The model under review builds one solid part; all positions refer to its coordinate system, in mm. A direction names the side the tool comes from. Coordinates: 2 decimals unless noted, no trailing zeros. Order: outer loops, then holes, each group sorted by start corner. A loop starts at its lowest first (then second) coordinate and runs counter-clockwise, first axis right, second up. Notation, with made-up numbers: (59, 7) -> (77, 7) arc R21 ccw to (77, 17) -> close; hole circle Ø9 at (86.25, 51). An arc over 180 degrees is marked (long way). Use one line per item in the form item = value. Start each with the question number.
(1) Take a section at B-B (x = 17.25). State the section outline as (y, z) points, then the cut area to 3 significant figures.
(2) Mouldability with a two-part tool opening along Y and no side actions: class faces 5 (the flat face through (5.5, 0, 22)), 6 (the flat face through (11, 13, 10)), 7 (the flat face through (13.933, 24.308, 10.07)) as +Y half, -Y half, draft (parallel to the pull), parting line (faces both ways), or undercut.
(3) Insertion check: pin 1 Ø4.5 at (y, z) = (-6, 20) entering from +X; pin 2 Ø5.5 at (y, z) = (19, 11.5) entering from -X; pin 3 Ø10 at (x, y) = (19, -15.5) entering from +Z. Each pin has a flat end and moves straight along its axis. Give the tip position at first contact, or say it passes through.
(4) Take a section at A-A (z = 8). State the section outline as (x, y) points, then the cut area to 3 significant figures.
(5) Wall thickness on line 1 along Y through (x, z) = (17, 9.5); line 2 along Y through (x, z) = (19.5, 5.25); line 3 along X through (y, z) = (-19.5, 11): over which ranges is each line inside the solid? List them lowest first.
(6) Take a section at C-C (z = 14). State the section outline as (x, y) points, then the cut area to 3 significant figures.
(7) Take a section at D-D (y = -11). State the section outline as (x, z) points, then the cut area to 3 significant figures.
(8) For faces 1 (the flat face through (5.5, -18, 10)), 2 (the flat face through (11, -13, 10)), 3 (the flat face through (14, 22, 5)), 4 (the flat face through (5.5, 18, 10)), list the 3-axis set-ups (+Z, -Z, +X, -X, +Y, -Y) from which the entire face can be reached by the end or side of a thin tool; tool diameter is ignored.
Autodesk Inventor part; units mm, degrees
ref_plane "YZ Plane" through (0, 0, 0) normal (1, 0, 0) x (0, 1, 0)
ref_plane "XZ Plane" through (0, 0, 0) normal (0, 1, 0) x (-1, 0, 0)
ref_plane "XY Plane" through (0, 0, 0) normal (0, 0, 1) x (1, 0, 0)
sketch "스케치1" plane through (0, 0, 0) normal (0, 0, 1) x (1, 0, 0)
  line L0 (0, 2.222) -> (0, -2.222)
  line L1 (0, -2.222) -> (22.6058, -12.8981)
  line L2 (22.6058, -12.8981) -> (22.6058, 12.8981)
  line L3 (22.6058, 12.8981) -> (0, 2.222)
  line L4 (0.5, 2.4581) -> (0.5, -2.4581)
  point P0 (0, 0)
  point P1 (0, 0)
  dimension "d0" = 25
  dimension "d1" = 115.28
  dimension "d2" = 115.28
  dimension "d3" = 4.444
  dimension "d4" = 0.5
extrude "돌출1" add sketch "스케치1" along normal blind 10 contours L3 L2 L1 L4
sketch "스케치2" plane through (0, 0, 10) normal (0, 0, 1) x (1, 0, 0)
  line L0 (0.5, 2.4581) -> (0.5, -2.4581)
  line L1 (0.5, -2.4581) -> (22.6058, -12.8981)
  line L2 (22.6058, -12.8981) -> (22.6058, 12.8981)
  line L3 (22.6058, 12.8981) -> (0.5, 2.4581)
  line L4 (0.5, 12.9643) -> (22.6058, 23.4042)
  line L5 (0.5, -12.9643) -> (22.6058, -23.4042)
  line L6 (22.6058, -23.4042) -> (22.6058, -12.8981)
  line L7 (22.6058, -12.8981) -> (22.6058, 12.8981)
  line L8 (22.6058, 23.4042) -> (22.6058, 12.8981)
  line L9 (0.5, 12.9643) -> (0.5, 2.4581)
  line L10 (0.5, 2.4581) -> (0.5, -2.4581)
  line L11 (0.5, -12.9643) -> (0.5, -2.4581)
  line L12 (22.6058, 12.8981) -> (0.5, 2.4581)
  line L13 (0.5, -2.4581) -> (22.6058, -12.8981)
  point P0 (0, 0)
  dimension "d23" = 9.5
  dimension "d24" = 9.5
extrude "돌출2" add sketch "스케치2" along normal blind 5
sketch "스케치3" plane through (0, 0, 15) normal (0, 0, 1) x (1, 0, 0)
  line L0 (22.6058, -23.4042) -> (22.6058, 23.4042)
  line L1 (22.6058, 23.4042) -> (0.5, 12.9643)
  line L2 (0.5, 12.9643) -> (0.5, -12.9643)
  line L3 (0.5, -12.9643) -> (22.6058, -23.4042)
  line L4 (22.6058, 23.4042) -> (0.5, 12.9643)
  line L5 (0.5, -12.9643) -> (22.6058, -23.4042)
  line L6 (5.5, 15.3256) -> (5.5, -15.3256)
  line L7 (0.5, 12.9643) -> (0.5, -12.9643)
  point P0 (0, 0)
  point P1 (5.5, -15.3256)
  dimension "d18" = 5
extrude "돌출3" add sketch "스케치3" along normal blind 15 contours L3 L2 L1 L6
sketch "스케치4" plane through (0, 0, 15) normal (0, 0, 1) x (1, 0, 0)
  line L0 (5.5, 15.3256) -> (5.5, -15.3256)
  line L1 (5.5, -15.3256) -> (22.6058, -23.4042)
  line L2 (22.6058, -23.4042) -> (22.6058, 23.4042)
  line L3 (22.6058, 23.4042) -> (5.5, 15.3256)
  line L4 (5.5, 15.3256) -> (5.5, -15.3256)
  line L5 (5.5, 15.3256) -> (5.5, 20.3256)
  line L6 (5.5, 20.3256) -> (22.6058, 28.4042)
  line L7 (22.6058, 12.8981) -> (22.6058, 23.4042)
  line L8 (22.6058, 28.4042) -> (22.6058, 23.4042)
  line L9 (5.5, -15.3256) -> (5.5, -20.3256)
  line L10 (5.5, -20.3256) -> (22.6058, -28.4042)
  line L11 (22.6058, -28.4042) -> (22.6058, -23.4042)
  line L12 (5.5, -15.3256) -> (22.6058, -23.4042)
  point P0 (0, 0)
  dimension "d19" = 5
  dimension "d20" = 5
extrude "돌출4" add sketch "스케치4" against normal blind 10 contours L5 L6 L8 L3 | L1 L11 L10 L9
properties part number "_3D 인쇄"
Findings:
q1.outline = (-25.87, 5) -> (-20.87, 5) -> (-20.87, 10) -> (-10.37, 10) -> (-10.37, 0) -> (10.37, 0) -> (10.37, 10) -> (20.87, 10) -> (20.87, 5) -> (25.87, 5) -> (25.87, 15) -> (-25.87, 15) -> close
q1.area = 516 mm²
q2.face_5 = draft
q2.face_6 = undercut
q2.face_7 = +Y half
q3.pin_1 = 5.5
q3.pin_2 = 5.5
q3.pin_3 = 15
q4.outline = (0.5, -2.46) -> (22.61, -12.9) -> (22.61, 12.9) -> (0.5, 2.46) -> close; (5.5, -20.33) -> (22.61, -28.4) -> (22.61, -23.4) -> (5.5, -15.33) -> close; (5.5, 15.33) -> (22.61, 23.4) -> (22.61, 28.4) -> (5.5, 20.33) -> close
q4.area = 511 mm²
q5.line_1 = -25.76 to -20.76, -10.25 to 10.25, 20.76 to 25.76
q5.line_2 = -26.94 to -21.94, -11.43 to 11.43, 21.94 to 26.94
q5.line_3 = 5.5 to 22.61
q6.outline = (0.5, -12.96) -> (5.5, -15.33) -> (5.5, -20.33) -> (22.61, -28.4) -> (22.61, 28.4) -> (5.5, 20.33) -> (5.5, 15.33) -> (0.5, 12.96) -> close
q6.area = 975 mm²
q7.outline = (0.5, 10) -> (18.59, 10) -> (18.59, 0) -> (22.61, 0) -> (22.61, 15) -> (5.5, 15) -> (5.5, 30) -> (0.5, 30) -> close
q7.area = 226 mm²
q8.face_1 = +Z, -Z, -X, -Y
q8.face_2 = -Z
q8.face_3 = -Z, +X, -X, +Y
q8.face_4 = +Z, -Z, -X, +Y
